Read the model definition and answer for the solid it produces. Units are mm, in the model's axes. Give positions to 0.01 mm unless a question says otherwise; leave off trailing zeros. Order: outer loops, then holes, each group sorted by start corner. A loop starts at its lowest first (then second) coordinate and runs counter-clockwise, first axis right, second up. Notation, with made-up numbers: (43.5, 36.25) - (85.5, 36.25) arc R32 cw to (85.5, 68.25) - close; hole circle Ø9 at (88.5, 72). An arc over 180 degrees is marked (long way). Write each question's results on one line, items separated by ' | '.
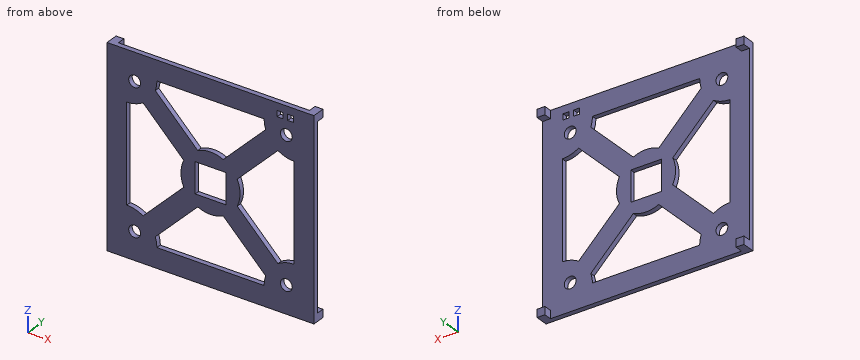
from build123d import *

# Parameters (mm, degrees)
SKETCH1_W           = 105
SKETCH1_H           = 100
BOSS_EXTRUDE1_DEPTH = 2.5
SKETCH3_W           = 4
SKETCH3_H           = 4
BOSS_EXTRUDE2_DEPTH = 4
SKETCH5_W           = 85
SKETCH5_H           = 80
CUT_EXTRUDE2_DEPTH  = 4
SKETCH6_R           = 15
BOSS_EXTRUDE3_DEPTH = 2.5
SKETCH7_W           = 15.5
SKETCH7_H           = 15.5
CUT_EXTRUDE3_DEPTH  = 2.5
BOSS_EXTRUDE4_DEPTH = 2.5
EXTRUDE_THIN2_DEPTH = 2.5
SKETCH10_R          = 3
CUT_EXTRUDE5_DEPTH  = 2.5
SKETCH11_W          = 3
SKETCH11_H          = 3
CUT_EXTRUDE6_DEPTH  = 2.5


with BuildPart() as part:
    # Sketch1 → Boss-Extrude1 (new body)
    with BuildSketch(Plane(origin=(0, 0, 0), x_dir=(1, 0, 0), z_dir=(0, 1, 0))):
        Rectangle(SKETCH1_W, SKETCH1_H)
    extrude(amount=BOSS_EXTRUDE1_DEPTH)

    # Sketch3 → Boss-Extrude2 (add)
    with BuildSketch(Plane(origin=(0, 2.5, 0), x_dir=(1, 0, 0), z_dir=(0, 1, 0))):
        with Locations((-50.5, 48)):
            Rectangle(SKETCH3_W, SKETCH3_H)
        with Locations((50.5, 48)):
            Rectangle(SKETCH3_W, SKETCH3_H)
        with Locations((50.5, -48)):
            Rectangle(SKETCH3_W, SKETCH3_H)
        with Locations((-50.5, -48)):
            Rectangle(SKETCH3_W, SKETCH3_H)
    extrude(amount=BOSS_EXTRUDE2_DEPTH)

    # Sketch5 → Cut-Extrude2 (cut)
    with BuildSketch(Plane(origin=(0, 2.5, 0), x_dir=(1, 0, 0), z_dir=(0, 1, 0))):
        Rectangle(SKETCH5_W, SKETCH5_H)
    extrude(amount=-CUT_EXTRUDE2_DEPTH, mode=Mode.SUBTRACT)

    # Sketch8 → Boss-Extrude4 (add)
    with BuildSketch(Plane(origin=(0, 2.5, 0), x_dir=(1, 0, 0), z_dir=(0, 1, 0))):
        with BuildLine():
            Line((-42.5, -40), (-27.220069463, -40))
            ThreePointArc((-27.220069463, -40), (-31.695457502, -29.195457502), (-42.5, -24.720069463))
            Line((-42.5, -24.720069463), (-42.5, -40))
        make_face()
        with BuildLine():
            ThreePointArc((-42.5, 24.720069463), (-31.695457502, 29.195457502), (-27.220069463, 40))
            Line((-27.220069463, 40), (-42.5, 40))
            Line((-42.5, 40), (-42.5, 24.720069463))
        make_face()
        with BuildLine():
            Line((42.5, 40), (27.220069463, 40))
            ThreePointArc((27.220069463, 40), (31.695457502, 29.195457502), (42.5, 24.720069463))
            Line((42.5, 24.720069463), (42.5, 40))
        make_face()
        with BuildLine():
            ThreePointArc((42.5, -24.720069463), (31.695457502, -29.195457502), (27.220069463, -40))
            Line((27.220069463, -40), (42.5, -40))
            Line((42.5, -40), (42.5, -24.720069463))
        make_face()
    extrude(amount=-BOSS_EXTRUDE4_DEPTH)



with BuildPart() as body_2:
    # Sketch6 → Boss-Extrude3 (new body)
    with BuildSketch(Plane(origin=(0, 2.5, 0), x_dir=(1, 0, 0), z_dir=(0, 1, 0))):
        with Locations(Location((0, 0, 0), (0, 0, 270))):
            Circle(SKETCH6_R)
    extrude(amount=-BOSS_EXTRUDE3_DEPTH)

    # Sketch7 → Cut-Extrude3 (cut)
    with BuildSketch(Plane(origin=(0, 2.5, 0), x_dir=(1, 0, 0), z_dir=(0, 1, 0))):
        Rectangle(SKETCH7_W, SKETCH7_H)
    extrude(amount=-CUT_EXTRUDE3_DEPTH, mode=Mode.SUBTRACT)


with BuildPart() as part_1:
    add(part.part)

    add(body_2.part)  # Extrude-Thin2 merges body 2
    # Sketch9 → Extrude-Thin2 (add)
    with BuildSketch(Plane(origin=(0, 2.5, 0), x_dir=(1, 0, 0), z_dir=(0, 1, 0))):
        Polygon((4.214466094, -11.285533906), (34.46870341, -41.539771222), (41.539771222, -34.46870341), (11.285533906, -4.214466094), align=None)
        Polygon((-11.285533906, -4.214466094), (-41.539771222, -34.46870341), (-34.46870341, -41.539771222), (-4.214466094, -11.285533906), align=None)
        Polygon((11.285533906, 4.214466094), (41.539771222, 34.46870341), (34.46870341, 41.539771222), (4.214466094, 11.285533906), align=None)
        Polygon((-4.214466094, 11.285533906), (-34.46870341, 41.539771222), (-41.539771222, 34.46870341), (-11.285533906, 4.214466094), align=None)
    extrude(amount=-EXTRUDE_THIN2_DEPTH)

    # Sketch10 → Cut-Extrude5 (cut)
    with BuildSketch(Plane(origin=(0, 2.5, 0), x_dir=(1, 0, 0), z_dir=(0, 1, 0))):
        with Locations(Location((38.5, 36, 0), (0, 0, 270))):
            Circle(SKETCH10_R)
        with Locations(Location((-38.5, 36, 0), (0, 0, 90))):
            Circle(SKETCH10_R)
        with Locations(Location((38.5, -36, 0), (0, 0, 90))):
            Circle(SKETCH10_R)
        with Locations(Location((-38.5, -36, 0), (0, 0, 270))):
            Circle(SKETCH10_R)
    extrude(amount=-CUT_EXTRUDE5_DEPTH, mode=Mode.SUBTRACT)

    # Sketch11 → Cut-Extrude6 (cut)
    with BuildSketch(Plane(origin=(0, 2.5, 0), x_dir=(1, 0, 0), z_dir=(0, 1, 0))):
        with Locations((40.657260224, -44.752137111)):
            Rectangle(SKETCH11_W, SKETCH11_H)
        with Locations((35.291405318, -44.752137111)):
            Rectangle(SKETCH11_W, SKETCH11_H)
    extrude(amount=-CUT_EXTRUDE6_DEPTH, mode=Mode.SUBTRACT)


solid = part_1.part
(1) Each of these flat-tipped pins is pushed along its axis until it touches: pin 1 (2 mm diameter, centred on x = -38, z = 28.5, fed in from +Y); pin 2 (1 mm diameter, centred on y = 4.5, z = 7, fed in from -X). Where does it stop, or does it pass through?
Conclusion:
pin 1: y = 2.5 | pin 2: through
(2) Section A-A (z = -37) is taken. Give the vertices of the cut face in (x, y).
Conclusion:
outline: (-52.5, 0) - (-41.33, 0) - (-41.33, 2.5) - (-52.5, 2.5) - close; (-35.67, 0) - (-27.52, 0) - (-27.52, 2.5) - (-35.67, 2.5) - close; (27.52, 0) - (35.67, 0) - (35.67, 2.5) - (27.52, 2.5) - close; (41.33, 0) - (52.5, 0) - (52.5, 2.5) - (41.33, 2.5) - close
(3) Consider probe 1 along X at (y, z) = (1, 36); probe 2 along X at (y, z) = (1.5, -2); probe 3 along Z at (x, y) = (6, 1). Determine where each line is inside the solid, lowest interval first. Write a range as [from, to].
Conclusion:
probe 1: [-52.5, -41.5], [-35.5, -27.75], [27.75, 35.5], [41.5, 52.5] | probe 2: [-52.5, -42.5], [-14.87, -7.75], [7.75, 14.87], [42.5, 52.5] | probe 3: [-50, -40], [-13.75, -7.75], [7.75, 13.75], [40, 50]
(4) Section B-B (y = 5.5) is taken. Give the vertices of the cut face in (x, z), plus the area to 3 significant figures.
Conclusion:
outline: (-52.5, -50) - (-48.5, -50) - (-48.5, -46) - (-52.5, -46) - close; (-52.5, 46) - (-48.5, 46) - (-48.5, 50) - (-52.5, 50) - close; (48.5, -50) - (52.5, -50) - (52.5, -46) - (48.5, -46) - close; (48.5, 46) - (52.5, 46) - (52.5, 50) - (48.5, 50) - close | area: 64.0 mm^2
